```python
from build123d import *

# Parameters (mm, degrees)
SKETCH_W        = 49
SKETCH_H        = 24
PAD_DEPTH       = 12
POCKET_DEPTH    = 12.001
SKETCH002_W     = 46
SKETCH002_H     = 21
POCKET001_DEPTH = 10
SKETCH003_W     = 8.5
SKETCH003_H     = 9.019632
POCKET002_DEPTH = 10
SKETCH004_W     = 14
SKETCH004_H     = 12
PAD001_DEPTH    = 10
SKETCH005_W     = 38
SKETCH005_H     = 12
PAD002_DEPTH    = 20
SKETCH006_R     = 4
POCKET003_DEPTH = 21
FILLET_R        = 2
FILLET001_R     = 2


with BuildPart() as part:
    # Sketch → Pad (new body)
    with BuildSketch(Plane.XY):
        Rectangle(SKETCH_W, SKETCH_H)
    extrude(amount=PAD_DEPTH)

    # Sketch001 (on Face6 of Pad) → Pocket (cut, through all)
    with BuildSketch(Plane.XY.offset(12)):
        with BuildLine():
            ThreePointArc((-10.5, 8), (-18.5, 0), (-10.5, -8))
            Line((-10.5, -8), (10.5, -8))
            ThreePointArc((10.5, -8), (18.5, 0), (10.5, 8))
            Line((10.5, 8), (-10.5, 8))
        make_face()
    extrude(amount=-POCKET_DEPTH, mode=Mode.SUBTRACT)

    # Sketch002 (on Face5 of Pocket) → Pocket001 (cut)
    with BuildSketch(Plane.XY.offset(12)):
        Rectangle(SKETCH002_W, SKETCH002_H)
    extrude(amount=-POCKET001_DEPTH, mode=Mode.SUBTRACT)

    # Sketch003 (on Face5 of Pocket001) → Pocket002 (cut)
    with BuildSketch(Plane.XY.offset(12)):
        with Locations((0, -11.77937)):
            Rectangle(SKETCH003_W, SKETCH003_H)
    extrude(amount=-POCKET002_DEPTH, mode=Mode.SUBTRACT)

    # Sketch004 (on Face6 of Pocket002) → Pad001 (join)
    with BuildSketch(Plane.XZ.offset(12)):
        with Locations((-12, 6)):
            Rectangle(SKETCH004_W, SKETCH004_H)
        with Locations((12, 6)):
            Rectangle(SKETCH004_W, SKETCH004_H)
    extrude(amount=PAD001_DEPTH)

    # Sketch005 (on Face30 of Pad001) → Pad002 (join)
    with BuildSketch(Plane.XZ.offset(22)):
        with Locations((0, 6)):
            Rectangle(SKETCH005_W, SKETCH005_H)
    extrude(amount=PAD002_DEPTH)

    # Sketch006 (on Face36 of Pad002) → Pocket003 (cut)
    with BuildSketch(Plane.XZ.offset(42)):
        with Locations((0, 6.129715)):
            Circle(SKETCH006_R)
    extrude(amount=-POCKET003_DEPTH, mode=Mode.SUBTRACT)

    # Fillet
    fillet_edges = [part.edges().sort_by_distance(p)[0] for p in [
        (24.5, -12, 6),
        (24.5, 12, 6),
        (-24.5, 12, 6),
        (-24.5, -12, 6),
    ]]
    fillet(fillet_edges, radius=FILLET_R)

    # Fillet001
    fillet001_edges = [part.edges().sort_by_distance(p)[0] for p in [
        (19, -32, 0),
        (-19, -32, 0),
        (19, -32, 12),
        (-19, -32, 12),
    ]]
    fillet(fillet001_edges, radius=FILLET001_R)


solid = part.part
```
The listing builds one solid part. Answer for the finished solid, in the listing's coordinates (mm). A direction names the side the tool comes from. Round coordinates to 2 decimals unless told otherwise and drop trailing zeros. Loops run counter-clockwise (first coordinate to the right, second up) from the corner with the lowest first, then second, coordinate; pieces in that order, holes last.
1) For a pull along Y with two mould halves and no side action, classify faces 5 (the face through (-23.9, 11.43, 6.08)), 6 (the face through (0, -12, 1)), 7 (the face through (24.5, 0, 6)) as released by +Y, released by -Y, zero draft, split by the parting line, or undercut.
Outcome:
face 5: released by +Y
face 6: undercut
face 7: zero draft
2) Consider line 1 (X direction, y = -9.5, z = 11.25); line 2 (Z direction, x = 0, y = -28.75); line 3 (Y direction, x = 18, z = 3.5). Determine where each line is inside the solid, lowest interval first.
Outcome:
line 1: x = -24.5 to -23, 23 to 24.5
line 2: z = 0 to 2.13, 10.13 to 12
line 3: y = -42 to -10.5, 10.5 to 12
3) A cutting plane is placed at A-A on y = 0. Determine the outline of the cut face in (x, z), plus the area to 3 significant figures.
Outcome:
outline: (-24.5, 0) - (-18.5, 0) - (-18.5, 2) - (-23, 2) - (-23, 12) - (-24.5, 12) - close; (18.5, 0) - (24.5, 0) - (24.5, 12) - (23, 12) - (23, 2) - (18.5, 2) - close
area: 54.0 mm2
4) For faces 1 (the face through (-18.43, -27.21, 0.6)), 2 (the face through (19, -27, 6)), 3 (the face through (-18.4, -26.79, 11.43)), 4 (the face through (-14, -10.5, 7)), determine the directions among +Z, -Z, +X, -X, +Y, -Y from which every point of the face is accessible in a straight line to the end or side of a thin tool.
Outcome:
face 1: -Z, -X, -Y
face 2: +Z, -Z, +X, -Y
face 3: +Z, -X, -Y
face 4: +Z
5) A cutting plane is placed at C-C on x = 21. Determine the outline of the cut face in (y, z), plus the area to 3 significant figures.
Outcome:
outline: (-12, 0) - (12, 0) - (12, 12) - (10.5, 12) - (10.5, 2) - (-10.5, 2) - (-10.5, 12) - (-12, 12) - close
area: 78.0 mm2
6) A cutting plane is placed at D-D on z = 8.5. Determine the outline of the cut face in (x, y).
Outcome:
outline: (-24.5, -10) arc R2 ccw to (-22.5, -12) - (-19, -12) - (-19, -42) - (-3.22, -42) - (-3.22, -22) - (-5, -22) - (-5, -12) - (-4.25, -12) - (-4.25, -10.5) - (-23, -10.5) - (-23, 10.5) - (23, 10.5) - (23, -10.5) - (4.25, -10.5) - (4.25, -12) - (5, -12) - (5, -22) - (3.22, -22) - (3.22, -42) - (19, -42) - (19, -12) - (22.5, -12) arc R2 ccw to (24.5, -10) - (24.5, 10) arc R2 ccw to (22.5, 12) - (-22.5, 12) arc R2 ccw to (-24.5, 10) - close
7) Given P1, Ø4, axis at y = -29.5, z = 7, coming from the -X side; P2, Ø6.5, axis at y = -28.5, z = 4, coming from the +X side; P3, Ø0.8, axis at y = -11.5, z = 9, coming from the +X side, each flat-ended and moving along its own axis, determine where each tip first touches the part or whether it passes through.
Outcome:
P1: stops at x = -19
P2: stops at x = 19
P3: stops at x = 24.17
8) A cutting plane is placed at B-B on x = -7. Determine the outline of the cut face in (y, z).
Outcome:
outline: (-42, 0) - (-8, 0) - (-8, 2) - (-10.5, 2) - (-10.5, 12) - (-42, 12) - close; (8, 0) - (12, 0) - (12, 12) - (10.5, 12) - (10.5, 2) - (8, 2) - close
